Could you check a few things on this model? Use its own coordinates, in mm. A direction names the side the tool comes from. Give positions to 0.01 mm unless a question says otherwise; leave off trailing zeros. Loops run counter-clockwise (first coordinate to the right, second up) from the corner with the lowest first, then second, coordinate; pieces in that order, holes last. Notation, with made-up numbers: (89, -26) - (125, -26) arc R14 cw to (125, -2) - close; hole circle Ø8 at (66.5, 51). An arc over 180 degrees is marked (long way). Write each question's results on one line, items separated by ' | '. Start each with the question number.
1) I want a section at C-C, the plane y = -23.5. Write out the boundary of the cut face in (x, z), and give its area (3 significant figures).
2) I want a section at D-D, the plane z = 10.75. Write out the boundary of the cut face in (x, y).
3) On a 3-axis mill with a long thin cutter (end or side, diameter ignored), from which of +Z, -Z, +X, -X, +Y, -Y can I reach the whole of each face in a straight line? I mean faces 1 (the face through (0, 0, 13)), 2 (the face through (-0.1, 20, -13.4)), 3 (the face through (0, 30, -3)), 4 (the face through (4, 0, 4)). Say none if no direction works.
4) I'm going to push flat-ended pins straight in: pin 1 (2 mm diameter, centred on x = 1.5, z = -3, fed in from +Y); pin 2 (2 mm diameter, centred on x = -2.5, y = -31.5, fed in from +Z); pin 3 (6.5 mm diameter, centred on x = 3.5, z = 1, fed in from +Y). Where does each tip first touch, or does it pass through?
5) If I drill on probe 1 along Y at (x, z) = (0, -5.6); probe 2 along Z at (x, y) = (0.75, 31); probe 3 along X at (y, z) = (14.5, 0.75), over which ranges is the centre line in solid material (lowest first)? Write a range as [from, to].
6) If we mould it in two halves opening along X, with no side actions, what happens to faces 5 (the face through (0, 30, -9)), 6 (the face through (4.6, 0.28, 12.14)), 7 (the face through (-5.361, 37.745, 6.042)), 8 (the face through (0, 20, -7))? For each: +X half, -X half, draft (parallel to the pull), parting line (faces both ways), or undercut.
7) I want a section at A-A, the plane y = 4. Count the separate pieces of the cut face and the enclosed holes in it, and give its area (3 significant figures).
from build123d import *

# Parameters (mm, degrees)
BOSS_EXTRUDE1_START  = -20
SKETCH1_W            = 15
SKETCH1_H            = 30
SKETCH1_W_2          = 2
SKETCH1_H_2          = 4
BOSS_EXTRUDE1_DEPTH  = 40
SKETCH2_W            = 15
SKETCH2_H            = 6
BOSS_EXTRUDE2_DEPTH  = 20
FILLET1_R            = 7.5
SKETCH3_R            = 1.5
CUT_EXTRUDE1_DEPTH   = 48.246693006
FILLET1_OF_MIRROR1_R = 7.5
FILLET2_R            = 3


with BuildPart() as part:
    # Sketch1 → Boss-Extrude1 (new body)
    with BuildSketch(Plane(origin=(0, 0, 0), x_dir=(1, 0, 0), z_dir=(0, 1, 0)).offset(BOSS_EXTRUDE1_START)):
        Rectangle(SKETCH1_W, SKETCH1_H)
        Polygon((-5.5, -13), (5.5, -13), (5.5, -4), (1.5, -4), (1.5, 4), (5.5, 4), (5.5, 13), (-5.5, 13), (-5.5, 4), (-1.5, 4), (-1.5, -4), (-5.5, -4), align=None, mode=Mode.SUBTRACT)
        with Locations((-4.5, 0)):
            Rectangle(SKETCH1_W_2, SKETCH1_H_2, mode=Mode.SUBTRACT)
        with Locations((4.5, 0)):
            Rectangle(SKETCH1_W_2, SKETCH1_H_2, mode=Mode.SUBTRACT)
    extrude(amount=BOSS_EXTRUDE1_DEPTH)

    # Sketch2 → Boss-Extrude2 (add)
    with BuildSketch(Plane.XZ.offset(20)):
        with Locations((0, 6)):
            Rectangle(SKETCH2_W, SKETCH2_H)
        with Locations((0, -6)):
            Rectangle(SKETCH2_W, SKETCH2_H)
    boss_extrude2 = extrude(amount=BOSS_EXTRUDE2_DEPTH)

    # Fillet1
    fillet1_edges = [part.edges().sort_by_distance(p)[0] for p in [
        (7.5, -40, 6),
        (7.5, -40, -6),
        (-7.5, -40, 6),
        (-7.5, -40, -6),
    ]]
    fillet(fillet1_edges, radius=FILLET1_R - 0.0001)  # a hair under: the kernel refuses the full size

    # Sketch3 → Cut-Extrude1 (cut, through all)
    with BuildSketch(Plane.XY.offset(9)):
        with Locations((0, -32.5)):
            Circle(SKETCH3_R)
    cut_extrude1 = extrude(amount=-CUT_EXTRUDE1_DEPTH, mode=Mode.SUBTRACT)

    # Mirror1: Boss-Extrude2, Cut-Extrude1 across plane
    add(boss_extrude2.mirror(Plane.ZX))
    add(cut_extrude1.mirror(Plane.ZX), mode=Mode.SUBTRACT)

    # Fillet1 of Mirror1
    fillet1_of_mirror1_edges = [part.edges().sort_by_distance(p)[0] for p in [
        (7.5, 40, 6),
        (7.5, 40, -6),
        (-7.5, 40, 6),
        (-7.5, 40, -6),
    ]]
    fillet(fillet1_of_mirror1_edges, radius=FILLET1_OF_MIRROR1_R - 0.0001)  # a hair under: the kernel refuses the full size

    # Fillet2
    fillet2_edges = [part.edges().sort_by_distance(p)[0] for p in [
        (5.5, 0, -13),
        (-5.5, 0, -13),
        (-5.5, 0, 13),
        (5.5, 0, 13),
        (7.5, 0, 15),
        (-7.5, 0, 15),
        (-7.5, 0, -15),
        (7.5, 0, -15),
    ]]
    fillet(fillet2_edges, radius=FILLET2_R)


solid = part.part
Answers:
1) outline: (-7.5, -9) - (7.5, -9) - (7.5, -3) - (-7.5, -3) - close; (-7.5, 3) - (7.5, 3) - (7.5, 9) - (-7.5, 9) - close | area: 180 mm2
2) outline: (-7.5, -20) - (-5.4, -20) - (-5.4, 20) - (-7.5, 20) - close; (5.4, -20) - (7.5, -20) - (7.5, 20) - (5.4, 20) - close
3) face 1: +Y, -Y | face 2: -Z, +X, -X, +Y | face 3: +X, -X, +Y | face 4: none
4) pin 1: stops at y = 39.98 | pin 2: stops at z = 9 | pin 3: stops at y = 39.94
5) probe 1: y = [-40, -34], [-31, -20], [20, 31], [34, 40] | probe 2: z = [-9, -3], [3, 9] | probe 3: x = [-7.5, -5.5], [-3.5, -1.5], [1.5, 3.5], [5.5, 7.5]
6) face 5: draft | face 6: undercut | face 7: -X half | face 8: undercut
7) separate pieces: 1 | enclosed holes: 3 | area: 212 mm2
